```python
from build123d import *

# Parameters (mm, degrees)
MODEL_R         = 1.65
EXTRUDE_1_DEPTH = 5


with BuildPart() as part:
    # Model → 凸台-拉伸1 (new body)
    with BuildSketch(Plane.XY):
        with BuildLine():
            Line((197.712050333, 317.514034213), (377.712050333, 317.514034213))
            ThreePointArc((377.712050333, 317.514034213), (384.783118145, 314.585102025), (387.712050333, 307.514034213))
            Line((387.712050333, 307.514034213), (387.712050333, 127.514034213))
            ThreePointArc((387.712050333, 127.514034213), (384.783118145, 120.442966401), (377.712050333, 117.514034213))
            Line((377.712050333, 117.514034213), (317.712050333, 117.514034213))
            Line((317.712050333, 117.514034213), (317.712050333, 237.514034213))
            Line((317.712050333, 237.514034213), (257.712050333, 237.514034213))
            Line((257.712050333, 237.514034213), (257.712050333, 117.514034213))
            Line((257.712050333, 117.514034213), (197.712050333, 117.514034213))
            ThreePointArc((197.712050333, 117.514034213), (190.640982521, 120.442966401), (187.712050333, 127.514034213))
            Line((187.712050333, 127.514034213), (187.712050333, 307.514034213))
            ThreePointArc((187.712050333, 307.514034213), (190.640982521, 314.585102025), (197.712050333, 317.514034213))
        make_face()
        with Locations((204.212050333, 236.014034213)):
            Circle(MODEL_R, mode=Mode.SUBTRACT)
        with Locations((197.712050333, 127.514034213)):
            Circle(MODEL_R, mode=Mode.SUBTRACT)
        with Locations((377.712050333, 127.514034213)):
            Circle(MODEL_R, mode=Mode.SUBTRACT)
        with Locations((197.712050333, 307.514034213)):
            Circle(MODEL_R, mode=Mode.SUBTRACT)
        with Locations((377.712050333, 307.514034213)):
            Circle(MODEL_R, mode=Mode.SUBTRACT)
        with Locations((241.212050333, 236.014034213)):
            Circle(MODEL_R, mode=Mode.SUBTRACT)
        with Locations((204.212050333, 199.014034213)):
            Circle(MODEL_R, mode=Mode.SUBTRACT)
        with Locations((241.212050333, 199.014034213)):
            Circle(MODEL_R, mode=Mode.SUBTRACT)
        with Locations((371.212050333, 236.014034213)):
            Circle(MODEL_R, mode=Mode.SUBTRACT)
        with Locations((334.212050333, 236.014034213)):
            Circle(MODEL_R, mode=Mode.SUBTRACT)
        with Locations((371.212050333, 199.014034213)):
            Circle(MODEL_R, mode=Mode.SUBTRACT)
        with Locations((334.212050333, 199.014034213)):
            Circle(MODEL_R, mode=Mode.SUBTRACT)
        with Locations((210.212050333, 290.514034213)):
            Circle(MODEL_R, mode=Mode.SUBTRACT)
        with Locations((224.212050333, 290.514034213)):
            Circle(MODEL_R, mode=Mode.SUBTRACT)
        with Locations((210.212050333, 274.514034213)):
            Circle(MODEL_R, mode=Mode.SUBTRACT)
        with Locations((224.212050333, 274.514034213)):
            Circle(MODEL_R, mode=Mode.SUBTRACT)
        with Locations((210.212050333, 144.514034213)):
            Circle(MODEL_R, mode=Mode.SUBTRACT)
        with Locations((210.212050333, 160.514034213)):
            Circle(MODEL_R, mode=Mode.SUBTRACT)
        with Locations((365.212050333, 290.514034213)):
            Circle(MODEL_R, mode=Mode.SUBTRACT)
        with Locations((351.212050333, 290.514034213)):
            Circle(MODEL_R, mode=Mode.SUBTRACT)
        with Locations((365.212050333, 274.514034213)):
            Circle(MODEL_R, mode=Mode.SUBTRACT)
        with Locations((351.212050333, 274.514034213)):
            Circle(MODEL_R, mode=Mode.SUBTRACT)
        with Locations((365.212050333, 144.514034213)):
            Circle(MODEL_R, mode=Mode.SUBTRACT)
        with Locations((365.212050333, 160.514034213)):
            Circle(MODEL_R, mode=Mode.SUBTRACT)
        with Locations((224.212050333, 144.514034213)):
            Circle(MODEL_R, mode=Mode.SUBTRACT)
        with Locations((224.212050333, 160.514034213)):
            Circle(MODEL_R, mode=Mode.SUBTRACT)
        with Locations((351.212050333, 144.514034213)):
            Circle(MODEL_R, mode=Mode.SUBTRACT)
        with Locations((351.212050333, 160.514034213)):
            Circle(MODEL_R, mode=Mode.SUBTRACT)
        with Locations((227.712050333, 246.514034213)):
            Circle(MODEL_R, mode=Mode.SUBTRACT)
        with Locations((217.712050333, 246.442167925)):
            Circle(MODEL_R, mode=Mode.SUBTRACT)
        with Locations((227.712050333, 188.514034213)):
            Circle(MODEL_R, mode=Mode.SUBTRACT)
        with Locations((217.712050333, 188.585900501)):
            Circle(MODEL_R, mode=Mode.SUBTRACT)
        Polygon((247.712050333, 142.514034213), (242.712050333, 142.514034213), (237.712050333, 142.514034213), (237.712050333, 162.514034213), (247.712050333, 162.514034213), align=None, mode=Mode.SUBTRACT)
        Polygon((327.712050333, 142.514034213), (332.712050333, 142.514034213), (337.712050333, 142.514034213), (337.712050333, 162.514034213), (327.712050333, 162.514034213), align=None, mode=Mode.SUBTRACT)
        Polygon((247.712050333, 292.514034213), (242.712050333, 292.514034213), (237.712050333, 292.514034213), (237.712050333, 272.514034213), (247.712050333, 272.514034213), align=None, mode=Mode.SUBTRACT)
        Polygon((327.712050333, 292.514034213), (332.712050333, 292.514034213), (337.712050333, 292.514034213), (337.712050333, 272.514034213), (327.712050333, 272.514034213), align=None, mode=Mode.SUBTRACT)
    extrude(amount=EXTRUDE_1_DEPTH)


solid = part.part
```
Can you work these out from the model? Positions are in its coordinate system, mm. A direction names the side the tool comes from. Give positions to 0.01 mm unless a question says otherwise; leave off trailing zeros. Write each loop counter-clockwise with the first axis right and the second up, starting at its lowest first coordinate (ties: lowest second). Pieces come first, ordered by that corner, then holes. Notation, with made-up numbers: (-28, -14.5) - (15, -14.5) arc R6 cw to (15, -5.5) - close; hole circle Ø8 at (61.5, 51.5). An arc over 180 degrees is marked (long way). Write item = value, one per line. Start each with the question number.
1. Imagine slicing it at A-A (y = 283.5). Please give me the cut outline in (x, z).
2. Imagine slicing it at C-C (z = 4.15). Count the separate pieces of the cut face and the enclosed holes in it, and give its area (3 significant figures).
3. On a 3-axis mill with a long thin cutter (end or side, diameter ignored), from which of +Z, -Z, +X, -X, +Y, -Y can I reach the whole of each face in a straight line? I mean faces 1 (the face through (243, 272.514, 2)), 2 (the face through (288, 237.514, 2)), 3 (the face through (384.86, 120.52, 2.46)). Say none if no direction works.
4. Thinking about a two-plate mould opening in Y: for faces 4 (the face through (190.719, 120.366, 2.465)), 5 (the face through (243, 142.514, 2)), 6 (the face through (190.564, 314.507, 2.465)), which applies, released by +Y, released by -Y, zero draft, split by the parting line, or undercut?
5. Imagine slicing it at D-D (x = 300.5). Please give me the cut outline in (y, z).
6. Please list where these lines run through material, in increasing order: line 1 (X direction, y = 155, z = 1.4); line 2 (Y direction, x = 330.5, z = 3.05); line 3 (Y direction, x = 198, z = 0.85).
7. For pin 1 (2.5 mm diameter, centred on x = 377.71, y = 127.51, fed in from +Z), with a flat end and sliding along its axis, tell me the tip position at first contact or that it passes through.
8. Imagine slicing it at B-B (y = 218). Please give me the cut outline in (x, z).
Worked answers:
q1.outline = (187.71, 0) - (237.71, 0) - (237.71, 5) - (187.71, 5) - close; (247.71, 0) - (327.71, 0) - (327.71, 5) - (247.71, 5) - close; (337.71, 0) - (387.71, 0) - (387.71, 5) - (337.71, 5) - close
q2.separate_pieces = 1
q2.enclosed_holes = 36
q2.area = 31,600 mm2
q3.face_1 = +Z, -Z
q3.face_2 = +Z, -Z, -Y
q3.face_3 = +Z, -Z, +X, -Y
q4.face_4 = released by -Y
q4.face_5 = undercut
q4.face_6 = released by +Y
q5.outline = (237.51, 0) - (317.51, 0) - (317.51, 5) - (237.51, 5) - close
q6.line_1 = 187.71 to 237.71, 247.71 to 257.71, 317.71 to 327.71, 337.71 to 387.71
q6.line_2 = 117.51 to 142.51, 162.51 to 272.51, 292.51 to 317.51
q6.line_3 = 117.51 to 125.89, 129.14 to 305.89, 309.14 to 317.51
q7.pin_1 = through
q8.outline = (187.71, 0) - (257.71, 0) - (257.71, 5) - (187.71, 5) - close; (317.71, 0) - (387.71, 0) - (387.71, 5) - (317.71, 5) - close
